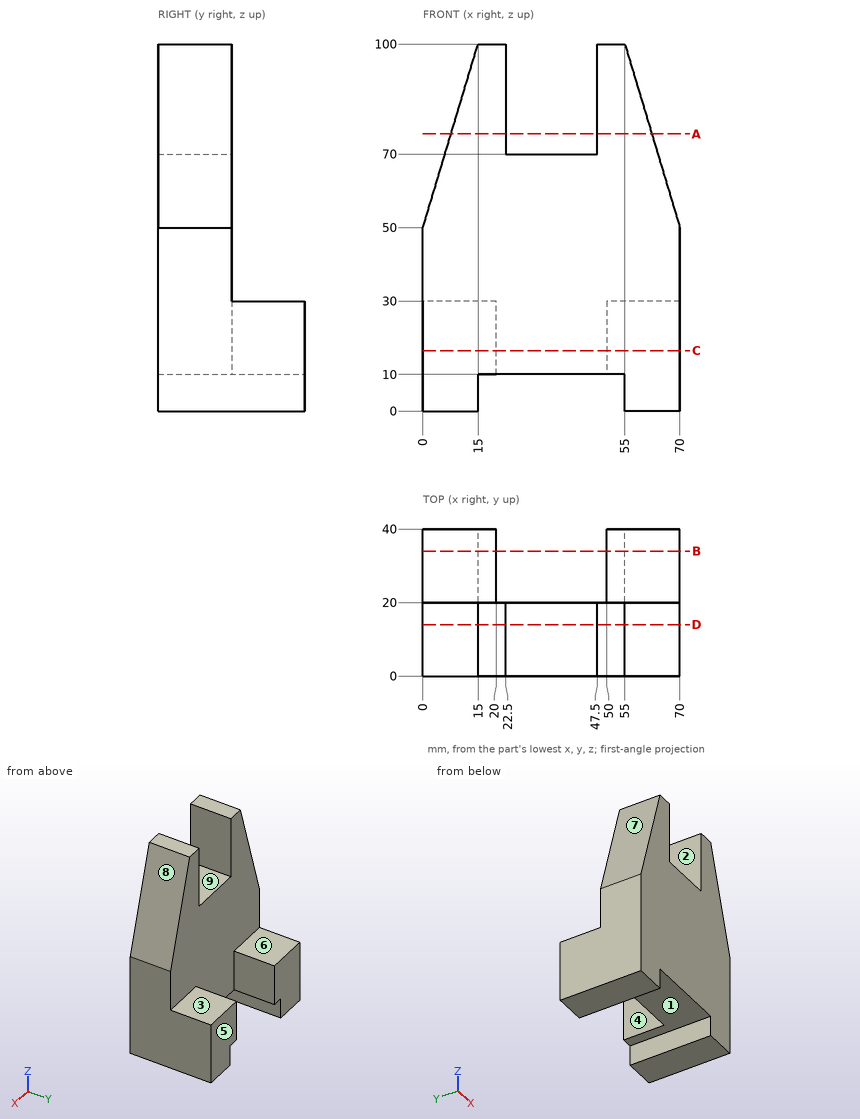
Geometry check sheet. Reference: drawing and pictorial views, mm from the part's lowest x, y, z. A direction names the side the tool comes from. Coordinates: 2 decimals unless noted, no trailing zeros. Order: outer loops, then holes, each group sorted by start corner. A loop starts at its lowest first (then second) coordinate and runs counter-clockwise, first axis right, second up. Notation, with made-up numbers: M 25,72.5 L 74,72.5 A25 ccw 74,108.5 Z; hole C 21,86.5 d4. An arc over 180 degrees is marked long. Write each question's results on one line, items separated by ' | '. Start each with the question number.
1. Cross-section at C-C on z = 16.5. Record the cut outline in (x, y).
2. Go/stop test with flat-tipped pins: P1, Ø10, axis at x = 10.5, y = 29, coming from the +Z side; P2, Ø20, axis at x = 29, y = 10.5, coming from the -Z side; P3, Ø10, axis at y = 17.5, z = 87, coming from the +X side. Record where each tip stops, or that it passes through.
3. Cross-section at A-A on z = 75.5. Record the cut outline in (x, y).
4. Access from +Z, -Z, +X, -X, +Y, -Y to the whole of each face (thin tool, end or side, straight path). Record for the marked faces 1, 2, 3, 4 and 5.
5. Mould release check, pull along X, two halves, no side actions. Record for the marked faces 6, 7, 8 and 9: +X half, -X half, draft (parallel to the pull), parting line (faces both ways), or undercut.
6. Cross-section at D-D on y = 14. Record the cut outline in (x, z).
7. Cross-section at B-B on y = 34. Record the cut outline in (x, z), and give its area (3 significant figures).
8. Material ranges on probe 1 along Z at (x, y) = (7, 25); probe 2 along Y at (x, z) = (20, 63); probe 3 along Z at (x, y) = (18.5, 36), recorded low to high.
Checks:
1) outline: M 0,0 L 70,0 L 70,40 L 50,40 L 50,20 L 20,20 L 20,40 L 0,40 Z
2) P1: stops at z = 30 | P2: stops at z = 10 | P3: stops at x = 60.4
3) outline: M 7.65,0 L 22.5,0 L 22.5,20 L 7.65,20 Z; M 47.5,0 L 62.35,0 L 62.35,20 L 47.5,20 Z
4) face 1: -Z, +Y, -Y | face 2: +Z, +Y, -Y | face 3: +Z, +X, -X, +Y | face 4: +Z, -Z, +Y | face 5: +Z, -Z, +X, -X, +Y
5) face 6: draft | face 7: -X half | face 8: +X half | face 9: undercut
6) outline: M 0,0 L 15,0 L 15,10 L 55,10 L 55,0 L 70,0 L 70,50 L 55,100 L 47.5,100 L 47.5,70 L 22.5,70 L 22.5,100 L 15,100 L 0,50 Z
7) outline: M 0,0 L 15,0 L 15,10 L 20,10 L 20,30 L 0,30 Z; M 50,10 L 55,10 L 55,0 L 70,0 L 70,30 L 50,30 Z | area: 1,100 mm²
8) probe 1: z = 0 to 30 | probe 2: y = 0 to 20 | probe 3: z = 10 to 30
